For this review, take the finished solid that the model builds, in its own axes (mm). Round coordinates to 2 decimals unless told otherwise and drop trailing zeros.
```python
from build123d import *

# Parameters (mm, degrees)
SKETCH1_R           = 2.0999999
BOSS_EXTRUDE1_DEPTH = 450


with BuildPart() as part:
    # Sketch1 → Boss-Extrude1 (new body)
    with BuildSketch(Plane(origin=(0, 0, 0), x_dir=(-1, 0, 0), z_dir=(0, 0, -1))):
        with BuildLine():
            Line((10, -19), (10, -13.3000005))
            ThreePointArc((10, -13.3000005), (9.912132034, -13.087868466), (9.7, -13.0000005))
            Line((9.7, -13.0000005), (7.999996324, -13.0000005))
            Line((7.999996324, -13.0000005), (7.999996324, -16.0000005))
            Line((7.999996324, -16.0000005), (7.0606365, -16.0000005))
            Line((7.0606365, -16.0000005), (4, -12.9393575))
            Line((4, -12.9393575), (4, -10.519615742))
            Line((4, -10.519615742), (3.7, -10.0000005))
            Line((3.7, -10.0000005), (4, -9.480385258))
            Line((4, -9.480385258), (4, -7.0606688))
            Line((4, -7.0606688), (7.06066257, -4.000000504))
            Line((7.06066257, -4.000000504), (7.999996324, -4.000000504))
            Line((7.999996324, -4.000000504), (7.999996324, -7.0000005))
            Line((7.999996324, -7.0000005), (9.7, -7.0000005))
            ThreePointArc((9.7, -7.0000005), (9.912132034, -6.912132534), (10, -6.7000005))
            Line((10, -6.7000005), (10, 6.7))
            ThreePointArc((10, 6.7), (9.912132034, 6.912132034), (9.7, 7))
            Line((9.7, 7), (7.999996324, 7))
            Line((7.999996324, 7), (7.999996324, 4))
            Line((7.999996324, 4), (7.060659, 4))
            Line((7.060659, 4), (4, 7.06066))
            Line((4, 7.06066), (4, 9.480384758))
            Line((4, 9.480384758), (3.7, 10))
            Line((3.7, 10), (4, 10.519615242))
            Line((4, 10.519615242), (4, 12.9393565))
            Line((4, 12.9393565), (7.060642, 16))
            Line((7.060642, 16), (7.999996324, 16))
            Line((7.999996324, 16), (7.999996324, 13))
            Line((7.999996324, 13), (9.7, 13))
            ThreePointArc((9.7, 13), (9.912132034, 13.087867966), (10, 13.3))
            Line((10, 13.3), (10, 19))
            ThreePointArc((10, 19), (9.707106781, 19.707106781), (9, 20))
            Line((9, 20), (3.3, 20))
            ThreePointArc((3.3, 20), (3.087867966, 19.912132034), (3, 19.7))
            Line((3, 19.7), (3, 17.999998284))
            Line((3, 17.999998284), (5.999998141, 17.999998284))
            Line((5.999998141, 17.999998284), (5.999998141, 17.060676141))
            Line((5.999998141, 17.060676141), (2.939333284, 13.999998284))
            Line((2.939333284, 13.999998284), (0.519636909, 13.999998284))
            Line((0.519636909, 13.999998284), (-1.716e-06, 13.699984784))
            Line((-1.716e-06, 13.699984784), (-0.519640341, 13.999998284))
            Line((-0.519640341, 13.999998284), (-2.939355716, 13.999998284))
            Line((-2.939355716, 13.999998284), (-6.000001716, 17.060658034))
            Line((-6.000001716, 17.060658034), (-6.000001716, 17.999998284))
            Line((-6.000001716, 17.999998284), (-3, 17.999998284))
            Line((-3, 17.999998284), (-3, 19.7))
            ThreePointArc((-3, 19.7), (-3.087867966, 19.912132034), (-3.3, 20))
            Line((-3.3, 20), (-9, 20))
            ThreePointArc((-9, 20), (-9.707106781, 19.707106781), (-10, 19))
            Line((-10, 19), (-10, 13.3))
            ThreePointArc((-10, 13.3), (-9.912132034, 13.087867966), (-9.7, 13))
            Line((-9.7, 13), (-8.000003676, 13))
            Line((-8.000003676, 13), (-8.000003676, 16))
            Line((-8.000003676, 16), (-7.060661, 16))
            Line((-7.060661, 16), (-4, 12.93933675))
            Line((-4, 12.93933675), (-4, 10.519615242))
            Line((-4, 10.519615242), (-3.7, 10))
            Line((-3.7, 10), (-4, 9.480384758))
            Line((-4, 9.480384758), (-4, 7.06068075))
            Line((-4, 7.06068075), (-7.060678, 4))
            Line((-7.060678, 4), (-8.000003676, 4))
            Line((-8.000003676, 4), (-8.000003676, 7))
            Line((-8.000003676, 7), (-9.7, 7))
            ThreePointArc((-9.7, 7), (-9.912132034, 6.912132034), (-10, 6.7))
            Line((-10, 6.7), (-10, -6.7000005))
            ThreePointArc((-10, -6.7000005), (-9.912132034, -6.912132534), (-9.7, -7.0000005))
            Line((-9.7, -7.0000005), (-8.000003676, -7.0000005))
            Line((-8.000003676, -7.0000005), (-8.000003676, -4.000000504))
            Line((-8.000003676, -4.000000504), (-7.06068236, -4.000000504))
            Line((-7.06068236, -4.000000504), (-4, -7.06068365))
            Line((-4, -7.06068365), (-4, -9.480385258))
            Line((-4, -9.480385258), (-3.7, -10.0000005))
            Line((-3.7, -10.0000005), (-4, -10.519615742))
            Line((-4, -10.519615742), (-4, -12.93934215))
            Line((-4, -12.93934215), (-7.06065685, -16.0000005))
            Line((-7.06065685, -16.0000005), (-8.000003676, -16.0000005))
            Line((-8.000003676, -16.0000005), (-8.000003676, -13.0000005))
            Line((-8.000003676, -13.0000005), (-9.7, -13.0000005))
            ThreePointArc((-9.7, -13.0000005), (-9.912132034, -13.087868466), (-10, -13.3000005))
            Line((-10, -13.3000005), (-10, -19))
            ThreePointArc((-10, -19), (-9.707106781, -19.707106781), (-9, -20))
            Line((-9, -20), (-3.3, -20))
            ThreePointArc((-3.3, -20), (-3.087867966, -19.912132034), (-3, -19.7))
            Line((-3, -19.7), (-3, -18.000001716))
            Line((-3, -18.000001716), (-6.000001716, -18.000001716))
            Line((-6.000001716, -18.000001716), (-6.000001716, -17.060664516))
            Line((-6.000001716, -17.060664516), (-2.939338216, -14.000001716))
            Line((-2.939338216, -14.000001716), (-0.519616958, -14.000001716))
            Line((-0.519616958, -14.000001716), (-1.716e-06, -13.700001716))
            Line((-1.716e-06, -13.700001716), (0.519613526, -14.000001716))
            Line((0.519613526, -14.000001716), (2.939316284, -14.000001716))
            Line((2.939316284, -14.000001716), (5.999998141, -17.060684359))
            Line((5.999998141, -17.060684359), (5.999998141, -18.000001716))
            Line((5.999998141, -18.000001716), (3, -18.000001716))
            Line((3, -18.000001716), (3, -19.7))
            ThreePointArc((3, -19.7), (3.087867966, -19.912132034), (3.3, -20))
            Line((3.3, -20), (9, -20))
            ThreePointArc((9, -20), (9.707106781, -19.707106781), (10, -19))
        make_face()
        with Locations((0, -10.0000005)):
            Circle(SKETCH1_R, mode=Mode.SUBTRACT)
        with Locations((0, 10)):
            Circle(SKETCH1_R, mode=Mode.SUBTRACT)
        with BuildLine():
            Line((7.999996324, 1.699995824), (7.999996324, -1.700003926))
            ThreePointArc((7.999996324, -1.700003926), (7.912128359, -1.91213596), (7.699996324, -2.000003926))
            Line((7.699996324, -2.000003926), (7.063600862, -2.000003926))
            ThreePointArc((7.063600862, -2.000003926), (6.94879664, -2.022827662), (6.85147763, -2.08786567))
            Line((6.85147763, -2.08786567), (2.939331324, -6.000003676))
            Line((2.939331324, -6.000003676), (-2.939335626, -6.000003676))
            Line((-2.939335626, -6.000003676), (-6.85148297, -2.087865332))
            ThreePointArc((-6.85148297, -2.087865332), (-6.948803597, -2.022827887), (-7.063608826, -2.000003926))
            Line((-7.063608826, -2.000003926), (-7.700003676, -2.000003926))
            ThreePointArc((-7.700003676, -2.000003926), (-7.91213571, -1.91213596), (-8.000003676, -1.700003926))
            Line((-8.000003676, -1.700003926), (-8.000003676, 1.699995824))
            ThreePointArc((-8.000003676, 1.699995824), (-7.91213571, 1.912127859), (-7.700003676, 1.999995824))
            Line((-7.700003676, 1.999995824), (-7.063603126, 1.999995824))
            ThreePointArc((-7.063603126, 1.999995824), (-6.948797876, 2.022820045), (-6.851477822, 2.087858478))
            Line((-6.851477822, 2.087858478), (-2.939339176, 5.999996324))
            Line((-2.939339176, 5.999996324), (2.939335324, 5.999996324))
            Line((2.939335324, 5.999996324), (6.85147158, 2.087857193))
            ThreePointArc((6.85147158, 2.087857193), (6.948790922, 2.02281871), (7.063595862, 1.999995824))
            Line((7.063595862, 1.999995824), (7.699996324, 1.999995824))
            ThreePointArc((7.699996324, 1.999995824), (7.912128359, 1.912127859), (7.999996324, 1.699995824))
        make_face(mode=Mode.SUBTRACT)
    extrude(amount=BOSS_EXTRUDE1_DEPTH)


solid = part.part
```
Q1. Take a section at A-A, the plane z = -130. Count the separate pieces of the cut face and the enclosed holes in it, plus the area to 3 significant figures.
Q2. Clearance check with flat-ended pins moving along their axes: pin 1 (6.5 mm diameter, centred on x = 0, y = -10, fed in from +Z); pin 2 (3 mm diameter, centred on x = -6, y = 11.5, fed in from +Z); pin 3 (1.9 mm diameter, centred on y = -8.5, z = -144.5, fed in from -X); pin 4 (6.5 mm diameter, centred on x = 0, z = -328.5, fed in from -Y). State where each tip first meets the part, or that it passes through.
Q3. Wall thickness on line 1 (Y direction, x = 8.25, z = -134); line 2 (X direction, y = 0, z = -361.5); line 3 (Y direction, x = 4.25, z = -199.5): over which ranges is each line inside the solid? List them lowest first.
Q4. Mouldability with a two-part tool opening along X and no side actions: class faces 1 (the face through (-10, 0, -222)), 2 (the face through (10, 0, -222)), 3 (the face through (5, 5, -450)) as +X half, -X half, draft (parallel to the pull), parting line (faces both ways), or undercut.
Working result:
1. separate pieces: 1
1. enclosed holes: 3
1. area: 324 mm2
2. pin 1: stops at z = 0
2. pin 2: passes through
2. pin 3: stops at x = -4
2. pin 4: stops at y = -20
3. line 1: y = -20 to -13, -7 to 7, 13 to 20
3. line 2: x = -10 to -8, 8 to 10
3. line 3: y = -20 to -18, -15.31 to -13.19, -6.81 to -4.69, 4.69 to 6.81, 13.19 to 15.31, 18 to 20
4. face 1: -X half
4. face 2: +X half
4. face 3: draft
